Could you check a few things on this model? Use its own coordinates, in mm. A direction names the side the tool comes from. Coordinates: 2 decimals unless noted, no trailing zeros. Write each loop counter-clockwise with the first axis right and the second up, starting at its lowest first coordinate (ties: lowest second). Pieces come first, ordered by that corner, then holes.
```python
from build123d import *

# Parameters (mm, degrees)
EXTRUDE_THIN1_DEPTH = 200
CUT_EXTRUDE1_DEPTH  = 364
FILLET1_R           = 20
SKETCH3_R           = 5
CUT_EXTRUDE2_DEPTH  = 417.173040934


with BuildPart() as part:
    # Sketch1 → Extrude-Thin1 (new, symmetric)
    with BuildSketch(Plane.XY):
        Polygon((-150, 60), (-150, 0), (210, 0), (210, 60), (200, 60), (200, 10), (-140, 10), (-140, 60), align=None)
    extrude(amount=EXTRUDE_THIN1_DEPTH, both=True)

    # Sketch2 → Cut-Extrude1 (cut)
    with BuildSketch(Plane(origin=(210, 0, 0), x_dir=(0, 0, -1), z_dir=(1, 0, 0))):
        with BuildLine():
            Line((40, 50), (140, 50))
            ThreePointArc((140, 50), (145, 45), (140, 40))
            Line((140, 40), (40, 40))
            ThreePointArc((40, 40), (35, 45), (40, 50))
        make_face()
    extrude(amount=-CUT_EXTRUDE1_DEPTH, mode=Mode.SUBTRACT)

    # Fillet1
    fillet1_edges = [part.edges().sort_by_distance(p)[0] for p in [
        (205, 60, 200),
        (-145, 60, 200),
        (205, 60, -200),
        (-145, 60, -200),
    ]]
    fillet(fillet1_edges, radius=FILLET1_R)

    # Sketch3 → Cut-Extrude2 (cut, through all)
    with BuildSketch(Plane.ZY.offset(150)):
        with Locations((180, 45)):
            Circle(SKETCH3_R)
    extrude(amount=-CUT_EXTRUDE2_DEPTH, mode=Mode.SUBTRACT)


solid = part.part
```
1. I want a section at B-B on z = -170. Please give me the cut outline in (x, y), plus the area to 3 significant figures.
Verdict:
outline: (-150, 0) - (210, 0) - (210, 60) - (200, 60) - (200, 10) - (-140, 10) - (-140, 60) - (-150, 60) - close
area: 4,600 mm2
2. I want a section at A-A on z = -77. Please give me the cut outline in (x, y).
Verdict:
outline: (-150, 0) - (210, 0) - (210, 40) - (200, 40) - (200, 10) - (-140, 10) - (-140, 40) - (-150, 40) - close; (-150, 50) - (-140, 50) - (-140, 60) - (-150, 60) - close; (200, 50) - (210, 50) - (210, 60) - (200, 60) - close
3. I want a section at C-C on x = 106.5. Please give me the cut outline in (y, z).
Verdict:
outline: (0, -200) - (10, -200) - (10, 200) - (0, 200) - close
4. Please list where these lines run through material, in increasing order: line 1 along X through (y, z) = (48.5, 134); line 2 along Y through (x, z) = (-144.5, 180); line 3 along Y through (x, z) = (106.5, 12).
Verdict:
line 1: x = -150 to -140, 200 to 210
line 2: y = 0 to 40, 50 to 60
line 3: y = 0 to 10
5. On a 3-axis mill with a long thin cutter (end or side, diameter ignored), from which of +Z, -Z, +X, -X, +Y, -Y can I reach the whole of each face in a straight line? I mean faces 5 (the face through (-145, 45, -145)), 6 (the face through (27, 0, 3)), 7 (the face through (32, 10, 3)). Say none if no direction works.
Verdict:
face 5: +X, -X
face 6: +Z, -Z, +X, -X, -Y
face 7: +Z, -Z, +Y
6. For pin 1 (6 mm diameter, centred on y = 45, z = 180, fed in from +X), with a flat end and sliding along its axis, tell me the tip position at first contact or that it passes through.
Verdict:
pin 1: passes through
7. If we mould it in two halves opening along Z, with no side actions, what happens to faces 1 (the face through (29.2, 9.7, -200)), 2 (the face through (-145, 40, -91)), 3 (the face through (-145, 50, -89)), 4 (the face through (-145, 60, 3))? For each: pulls with the +Z half, pulls with the -Z half, needs draft (parallel to the pull), parting line crosses it, or undercut.
Verdict:
face 1: pulls with the -Z half
face 2: undercut
face 3: undercut
face 4: needs draft
